Can you work these out from the drawing? Everything is in mm from the part's minimum corner. A direction names the side the tool comes from. Coordinates: 2 decimals unless noted, no trailing zeros. Write each loop counter-clockwise with the first axis right and the second up, starting at its lowest first coordinate (ties: lowest second). Pieces come first, ordered by that corner, then holes.
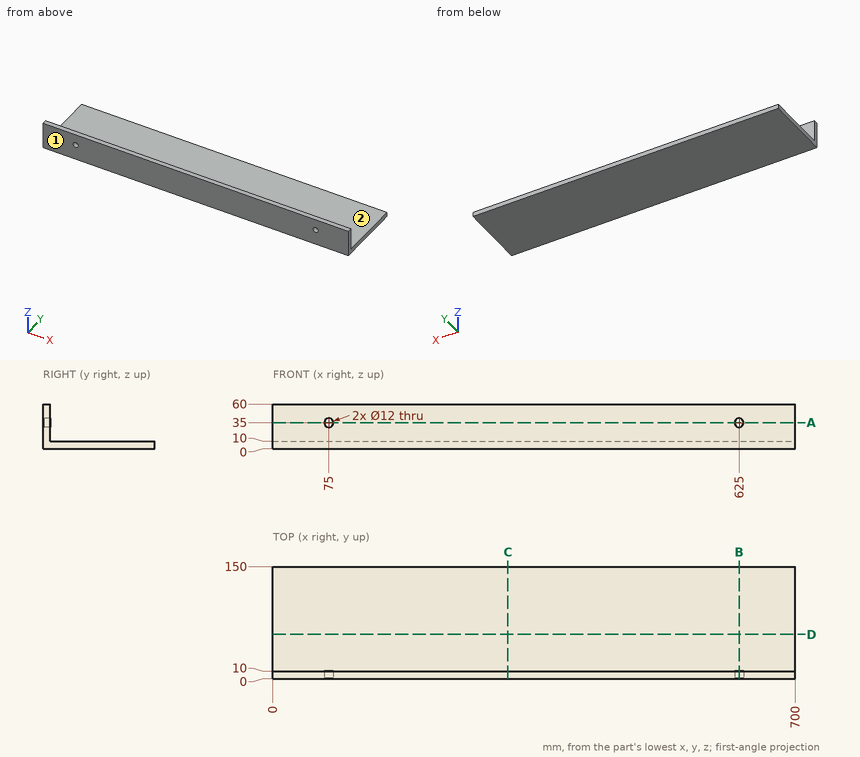
1. For pin 1 Ø15 at (x, z) = (364, 44) entering from +Y, with a flat end and sliding along its axis, tell me the tip position at first contact or that it passes through.
2. If I drill on line 1 (X direction, y = 7.5, z = 35); line 2 (Z direction, x = 625, y = 3); line 3 (Y direction, x = 670.5, z = 19.5), over which ranges is the centre line in solid material (lowest first)?
3. On a 3-axis mill with a long thin cutter (end or side, diameter ignored), from which of +Z, -Z, +X, -X, +Y, -Y can I reach the whole of each face in a straight line? I mean the marked faces 1 and 2. Say none if no direction works.
4. I want a section at C-C (x = 315). List the corners of the cut face in (y, z) for me, then the cut area to 3 significant figures.
5. I want a section at A-A (z = 35). List the corners of the cut face in (x, y) for me.
6. I want a section at B-B (x = 625). List the corners of the cut face in (y, z) for me, then the cut area to 3 significant figures.
7. I want a section at D-D (y = 59.5). List the corners of the cut face in (x, z) for me.
Response values:
1. pin 1: stops at y = 10
2. line 1: x = 0 to 69, 81 to 619, 631 to 700
2. line 2: z = 0 to 29, 41 to 60
2. line 3: y = 0 to 10
3. face 1: +Z, -Z, +X, -X, -Y
3. face 2: +Z, +X, -X, +Y
4. outline: (0, 0) - (150, 0) - (150, 10) - (10, 10) - (10, 60) - (0, 60) - close
4. area: 2,000 mm2
5. outline: (0, 0) - (69, 0) - (69, 10) - (0, 10) - close; (81, 0) - (619, 0) - (619, 10) - (81, 10) - close; (631, 0) - (700, 0) - (700, 10) - (631, 10) - close
6. outline: (0, 0) - (150, 0) - (150, 10) - (10, 10) - (10, 29) - (0, 29) - close; (0, 41) - (10, 41) - (10, 60) - (0, 60) - close
6. area: 1,880 mm2
7. outline: (0, 0) - (700, 0) - (700, 10) - (0, 10) - close
